CAD build for the part. Positions are in the model's coordinates, mm. Face numbers are marked on the shaded views. A direction names the side the tool comes from. Coordinates: 2 decimals unless noted, no trailing zeros. Write each loop counter-clockwise with the first axis right and the second up, starting at its lowest first coordinate (ties: lowest second). Pieces come first, ordered by that corner, then holes. Notation, with made-up numbers: (3.25, 58) -> (36.25, 58) arc R25 cw to (36.25, 87) -> close; hole circle Ø7 at (14, -9). An arc over 180 degrees is marked (long way). Answer as CSV lines item,"result".
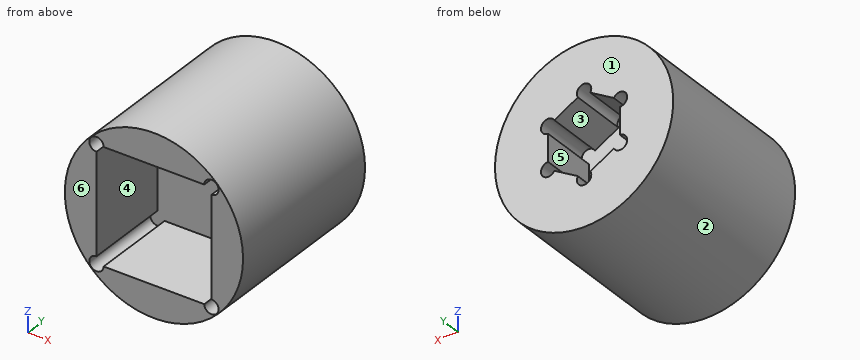
```python
from build123d import *

# Parameters (mm, degrees)
SKETCH3_R           = 19.685
BOSS_EXTRUDE1_DEPTH = 19.05
SKETCH4_R           = 1.5875
SKETCH4_W           = 25.4
SKETCH4_H           = 25.4
CUT_EXTRUDE1_DEPTH  = 19.05
SKETCH5_R           = 1.5875
CUT_EXTRUDE2_DEPTH  = 12.7


with BuildPart() as part:
    # Sketch3 → Boss-Extrude1 (new body, symmetric)
    with BuildSketch(Plane(origin=(0, 0, 0), x_dir=(1, 0, 0), z_dir=(0, 1, 0))):
        Circle(SKETCH3_R)
    extrude(amount=BOSS_EXTRUDE1_DEPTH, both=True)

    # Sketch4 → Cut-Extrude1 (cut)
    with BuildSketch(Plane.XZ.offset(19.05)):
        with Locations((12.7, -12.7)):
            Circle(SKETCH4_R)
        with Locations((-12.7, -12.7)):
            Circle(SKETCH4_R)
        with Locations((-12.7, 12.7)):
            Circle(SKETCH4_R)
        with Locations((12.7, 12.7)):
            Circle(SKETCH4_R)
        Rectangle(SKETCH4_W, SKETCH4_H)
    extrude(amount=-CUT_EXTRUDE1_DEPTH, mode=Mode.SUBTRACT)

    # Sketch5 → Cut-Extrude2 (cut)
    with BuildSketch(Plane(origin=(0, 19.05, 0), x_dir=(1, 0, 0), z_dir=(0, 1, 0))):
        with Locations((7.9375, 4.582717762)):
            Circle(SKETCH5_R)
        with Locations((0, 9.165435523)):
            Circle(SKETCH5_R)
        with Locations((-7.9375, 4.582717762)):
            Circle(SKETCH5_R)
        with Locations((-7.9375, -4.582717762)):
            Circle(SKETCH5_R)
        with Locations((0, -9.165435523)):
            Circle(SKETCH5_R)
        with Locations((7.9375, -4.582717762)):
            Circle(SKETCH5_R)
        Polygon((7.9375, 4.582717762), (0, 9.165435523), (-7.9375, 4.582717762), (-7.9375, -4.582717762), (0, -9.165435523), (7.9375, -4.582717762), align=None)
        with BuildLine():
            ThreePointArc((-6.35, -4.582717762), (-6.814967985, -3.460185747), (-7.9375, -2.995217762))
            Line((-7.9375, -2.995217762), (-7.9375, -4.582717762))
            Line((-7.9375, -4.582717762), (-6.562684671, -5.376467762))
            ThreePointArc((-6.562684671, -5.376467762), (-6.404092751, -4.993592996), (-6.35, -4.582717762))
        make_face()
        with BuildLine():
            Line((-7.9375, -4.582717762), (-7.9375, -2.995217762))
            ThreePointArc((-7.9375, -2.995217762), (-9.312315329, -5.376467762), (-6.562684671, -5.376467762))
            Line((-6.562684671, -5.376467762), (-7.9375, -4.582717762))
        make_face()
        with BuildLine():
            ThreePointArc((1.374815329, -8.371685523), (0, -7.577935523), (-1.374815329, -8.371685523))
            Line((-1.374815329, -8.371685523), (0, -9.165435523))
            Line((0, -9.165435523), (1.374815329, -8.371685523))
        make_face()
        with BuildLine():
            Line((0, -9.165435523), (-1.374815329, -8.371685523))
            ThreePointArc((-1.374815329, -8.371685523), (-0.410875234, -10.698842773), (1.5875, -9.165435523))
            ThreePointArc((1.5875, -9.165435523), (1.533407249, -8.754560289), (1.374815329, -8.371685523))
            Line((1.374815329, -8.371685523), (0, -9.165435523))
        make_face()
        with BuildLine():
            ThreePointArc((9.525, -4.582717762), (9.060032015, -3.460185747), (7.9375, -2.995217762))
            Line((7.9375, -2.995217762), (7.9375, -4.582717762))
            Line((7.9375, -4.582717762), (6.562684671, -5.376467762))
            ThreePointArc((6.562684671, -5.376467762), (8.348375234, -6.116125011), (9.525, -4.582717762))
        make_face()
        with BuildLine():
            Line((7.9375, -4.582717762), (7.9375, -2.995217762))
            ThreePointArc((7.9375, -2.995217762), (6.562684671, -3.788967762), (6.562684671, -5.376467762))
            Line((6.562684671, -5.376467762), (7.9375, -4.582717762))
        make_face()
        with BuildLine():
            ThreePointArc((9.525, 4.582717762), (8.348375234, 6.116125011), (6.562684671, 5.376467762))
            Line((6.562684671, 5.376467762), (7.9375, 4.582717762))
            Line((7.9375, 4.582717762), (7.9375, 2.995217762))
            ThreePointArc((7.9375, 2.995217762), (9.060032015, 3.460185747), (9.525, 4.582717762))
        make_face()
        with BuildLine():
            Line((7.9375, 4.582717762), (6.562684671, 5.376467762))
            ThreePointArc((6.562684671, 5.376467762), (6.562684671, 3.788967762), (7.9375, 2.995217762))
            Line((7.9375, 2.995217762), (7.9375, 4.582717762))
        make_face()
        with BuildLine():
            Line((1.374815329, 8.371685523), (0, 9.165435523))
            Line((0, 9.165435523), (-1.374815329, 8.371685523))
            ThreePointArc((-1.374815329, 8.371685523), (0, 7.577935523), (1.374815329, 8.371685523))
        make_face()
        with BuildLine():
            Line((-1.374815329, 8.371685523), (0, 9.165435523))
            Line((0, 9.165435523), (1.374815329, 8.371685523))
            ThreePointArc((1.374815329, 8.371685523), (1.533407249, 8.754560289), (1.5875, 9.165435523))
            ThreePointArc((1.5875, 9.165435523), (-0.410875234, 10.698842773), (-1.374815329, 8.371685523))
        make_face()
        with BuildLine():
            ThreePointArc((-6.35, 4.582717762), (-6.404092751, 4.993592996), (-6.562684671, 5.376467762))
            Line((-6.562684671, 5.376467762), (-7.9375, 4.582717762))
            Line((-7.9375, 4.582717762), (-7.9375, 2.995217762))
            ThreePointArc((-7.9375, 2.995217762), (-6.814967985, 3.460185747), (-6.35, 4.582717762))
        make_face()
        with BuildLine():
            Line((-7.9375, 4.582717762), (-6.562684671, 5.376467762))
            ThreePointArc((-6.562684671, 5.376467762), (-9.312315329, 5.376467762), (-7.9375, 2.995217762))
            Line((-7.9375, 2.995217762), (-7.9375, 4.582717762))
        make_face()
    extrude(amount=-CUT_EXTRUDE2_DEPTH, mode=Mode.SUBTRACT)


solid = part.part
```
Item 1: Wall check: line 1 (Z direction, x = -5, y = -6); line 2 (Z direction, x = -0.5, y = -16.5); line 3 (Z direction, x = -14, y = -9). Give the ranges that are in metal, low to high. Write a range as from..to.
Answer below:
line 1,"z = -19.04..-12.7, 12.7..19.04"
line 2,"z = -19.68..-12.7, 12.7..19.68"
line 3,"z = -13.84..-13.61, -11.79..11.79, 13.61..13.84"
Item 2: Flat gauge pins, fed straight in: pin 1 (14.5 mm diameter, centred on x = -5, z = 6.5, fed in from -Y); pin 2 (9.5 mm diameter, centred on x = 0, y = -13.5, fed in from -Z) (3 decimals); pin 3 (5.5 mm diameter, centred on x = -0.5, z = 4.5, fed in from +Y); pin 4 (2 mm diameter, centred on y = -2.5, z = -9.5, fed in from +X). Where does each tip first touch, or does it go through?
Answer below:
pin 1,"stops at y = -19.05"
pin 2,"stops at z = -19.685"
pin 3,"stops at y = 6.35"
pin 4,"stops at x = 17.76"
Item 3: 3-axis set-ups, long thin cutter, end or side, ignore diameter. For the marked faces 4, 5 and 6: which of +Z, -Z, +X, -X, +Y, -Y reach the whole face in a straight line?
Answer below:
face 4,"-Y"
face 5,"+Y"
face 6,"+Z, -Z, +X, -X, -Y"
Item 4: Saw through at C-C on x = 3. Give the cut face in (y, z), and give its area (3 significant figures).
Answer below:
outline,"(-19.05, -19.46) -> (19.05, -19.46) -> (19.05, -7.43) -> (6.35, -7.43) -> (6.35, 7.43) -> (19.05, 7.43) -> (19.05, 19.46) -> (-19.05, 19.46) -> (-19.05, 12.7) -> (0, 12.7) -> (0, -12.7) -> (-19.05, -12.7) -> close"
area,"810 mm2"
Item 5: Two-plate mould, pull along Z, no slides. Class the marked faces 1, 2 and 3: pulls with the +Z half, pulls with the -Z half, needs draft (parallel to the pull), parting line crosses it, or undercut.
Answer below:
face 1,"needs draft"
face 2,"parting line crosses it"
face 3,"undercut"
Item 6: Saw through at D-D on y = -10. Give the cut face in (x, z) (1 decimal).
Answer below:
outline,"circle Ø39.4 at (0, 0); hole (-12.7, -11.1) arc R1.6 ccw (long way) to (-11.1, -12.7) -> (11.1, -12.7) arc R1.6 ccw (long way) to (12.7, -11.1) -> (12.7, 11.1) arc R1.6 ccw (long way) to (11.1, 12.7) -> (-11.1, 12.7) arc R1.6 ccw (long way) to (-12.7, 11.1) -> close"
Item 7: Saw through at A-A on y = 10. Give the cut face in (x, z) (1 decimal).
Answer below:
outline,"circle Ø39.4 at (0, 0); hole (-7.9, -3) arc R1.6 ccw (long way) to (-6.6, -5.4) -> (-1.4, -8.4) arc R1.6 ccw (long way) to (1.4, -8.4) -> (6.6, -5.4) arc R1.6 ccw (long way) to (7.9, -3) -> (7.9, 3) arc R1.6 ccw (long way) to (6.6, 5.4) -> (1.4, 8.4) arc R1.6 ccw (long way) to (-1.4, 8.4) -> (-6.6, 5.4) arc R1.6 ccw (long way) to (-7.9, 3) -> close"
